```python
from build123d import *

# Parameters (mm, degrees)
F0_W      = 61.827414
F0_H      = 102.335028
F1_DEPTH  = 5
F2_W      = 5.862944
F2_H      = 102.335028
F2_W_2    = 7.728428
F3_DEPTH  = 10
F4_W      = 61.827414
F4_H      = 9.661161
F5_DEPTH  = 5
F6_W      = 61.827414
F6_H      = 4.830581
F7_DEPTH  = 8
F8_W      = 48.236042
F8_H      = 22.642768
F9_DEPTH  = 5
F10_W     = 48.06122
F10_H     = 23.24395
F11_DEPTH = 2
F13_DEPTH = 8


with BuildPart() as f1:
    # F0 (on Top) → F1 (new body)
    with BuildSketch(Plane.XY):
        Rectangle(F0_W, F0_H)
        Polygon((-30.913707, -51.167514), (-30.913707, 51.167514), (-54.365486, 25.317261), align=None)
        Polygon((52.766502, 25.317261), (30.913707, 51.167514), (30.913707, -51.167514), align=None)
    extrude(amount=F1_DEPTH)

    # F2 (on face) → F3 (join)
    with BuildSketch(Plane.XY.offset(5)):
        with Locations((-27.982235, 0)):
            Rectangle(F2_W, F2_H)
        with Locations((27.049493, 0)):
            Rectangle(F2_W_2, F2_H)
    extrude(amount=F3_DEPTH)

    # F4 (on face) → F5 (join)
    with BuildSketch(Plane(origin=(0, 0, 0), x_dir=(1, 0, 0), z_dir=(0, 0, -1))):
        with Locations((0, -55.998094)):
            Rectangle(F4_W, F4_H)
    extrude(amount=-F5_DEPTH)

    # F6 (on face) → F7 (join)
    with BuildSketch(Plane.XY.offset(5)):
        with Locations((0, 58.413384)):
            Rectangle(F6_W, F6_H)
    extrude(amount=F7_DEPTH)

    # F8 (on face) → F9 (cut)
    with BuildSketch(Plane.XY.offset(5)):
        with Locations((-0.932742, -20.754081)):
            Rectangle(F8_W, F8_H)
    extrude(amount=-F9_DEPTH, mode=Mode.SUBTRACT)

    # F10 (on face) → F11 (join)
    with BuildSketch(Plane.XY.offset(15)):
        with Locations((-1.020153, -20.942758)):
            Rectangle(F10_W, F10_H)
    extrude(amount=-F11_DEPTH)

    # F12 (on face) → F13 (join)
    with BuildSketch(Plane(origin=(0, 0, 0), x_dir=(1, 0, 0), z_dir=(0, 0, -1))):
        with BuildLine():
            ThreePointArc((-41.82278, -18.125845), (-49.30103, -25.974858), (-41.573606, -33.578683))
            Line((-41.573606, -33.578683), (-41.82278, -18.125845))
        make_face()
        with BuildLine():
            ThreePointArc((41.573606, -33.578683), (49.30103, -25.974858), (41.82278, -18.125845))
            Line((41.82278, -18.125845), (41.573606, -33.578683))
        make_face()
    extrude(amount=F13_DEPTH)


solid = f1.part
```
Source: CAD feature listing. Evaluate the final solid. Frame: model axes, mm. A direction names the side the tool comes from. Round coordinates to 2 decimals unless told otherwise and drop trailing zeros. Loops run counter-clockwise (first coordinate to the right, second up) from the corner with the lowest first, then second, coordinate; pieces in that order, holes last.
1. Access query for faces 4 (the flat face through (-30.914, -1, 10)), 5 (the flat face through (-25.051, -1, 9)), 6 (the flat face through (0, 55.998, 9)), 7 (the flat face through (0, 58, 13)), 8 (the cylindrical face through (-49.3, 25.8, -3.9)). Directions: +Z, -Z, +X, -X, +Y, -Y. A direction counts if a zero-diameter tool reaches every point of the face in a straight line with its end or side. Return the directions, or none.
2. Mould query, pull axis Y, two halves, no side actions, for faces 1 (the flat face through (27, 51.168, 10)), 2 (the flat face through (-1, -42, 5)), 3 (the cylindrical face through (49.296, 26.143, -3.944)). Classes: released by +Y, released by -Y, zero draft, split by the parting line, or undercut.
3. Ray query, L1, parallel to X at y = 0.5, z = 10.5; L2, parallel to Y at x = -13, z = 9; L3, parallel to Z at x = -25.5, y = -34. Return the intervals inside material, ascending.
4. Section query A-A on x = 1. Output: boundary loops of the cut face in (y, z), and give its area (3 significant figures).
5. Section query C-C on y = -30. Output: boundary loops of the cut face in (x, z), and give its area (3 significant figures).
6. Section query B-B on z = 7.25. Output: boundary loops of the cut face in (x, y).
7. Section query D-D on x = -28.5. Output: boundary loops of the cut face in (y, z).
8. Contact query for flat-ended pins moving along their axis: pin 1 (3 mm diameter, centred on x = 36.5, z = 1, fed in from +Y); pin 2 (12 mm diameter, centred on x = -27, y = 38.5, fed in from -Z); pin 3 (5.5 mm diameter, centred on x = -3.5, y = -43, fed in from +Z); pin 4 (1.5 mm diameter, centred on x = -38, z = -2, fed in from +Y). Output: stop coordinate, or through.
Answers below:
1. face 4: +Z, -X, +Y, -Y
1. face 5: none
1. face 6: +Z, +X, -X
1. face 7: +Z, +X, -X, +Y
1. face 8: -Z, -X
2. face 1: undercut
2. face 2: zero draft
2. face 3: split by the parting line
3. L1: x = -30.91 to -25.05, 23.19 to 30.91
3. L2: y = 56 to 60.83
3. L3: z = 0 to 15
4. outline: (-51.17, 0) - (-32.08, 0) - (-32.08, 5) - (-51.17, 5) - close; (-32.56, 13) - (-9.32, 13) - (-9.32, 15) - (-32.56, 15) - close; (-9.43, 0) - (60.83, 0) - (60.83, 13) - (56, 13) - (56, 5) - (-9.43, 5) - close
4. area: 532 mm2
5. outline: (-37.4, 0) - (-25.05, 0) - (-25.05, 13) - (23.01, 13) - (23.01, 15) - (-30.91, 15) - (-30.91, 5) - (-37.4, 5) - close; (23.19, 0) - (36.96, 0) - (36.96, 5) - (30.91, 5) - (30.91, 15) - (23.19, 15) - close
5. area: 363 mm2
6. outline: (-30.91, -51.17) - (-25.05, -51.17) - (-25.05, 51.17) - (-30.91, 51.17) - close; (-30.91, 56) - (30.91, 56) - (30.91, 60.83) - (-30.91, 60.83) - close; (23.19, -51.17) - (30.91, -51.17) - (30.91, 51.17) - (23.19, 51.17) - close
7. outline: (-51.17, 0) - (60.83, 0) - (60.83, 13) - (56, 13) - (56, 5) - (51.17, 5) - (51.17, 15) - (-51.17, 15) - close
8. pin 1: stops at y = 46.33
8. pin 2: stops at z = 0
8. pin 3: stops at z = 5
8. pin 4: passes through
